Could you check a few things on this model? Use its own coordinates, in mm. Face numbers are marked on the shaded views. A direction names the side the tool comes from. Round coordinates to 2 decimals unless told otherwise and drop trailing zeros. Loops run counter-clockwise (first coordinate to the right, second up) from the corner with the lowest first, then second, coordinate; pieces in that order, holes last. Notation, with made-up numbers: (55, 45.25) -> (60, 45.25) arc R14 cw to (60, 67.25) -> close; hole circle Ø5 at (44, -31.75). An arc over 180 degrees is marked (long way). One line per item, written item: value.
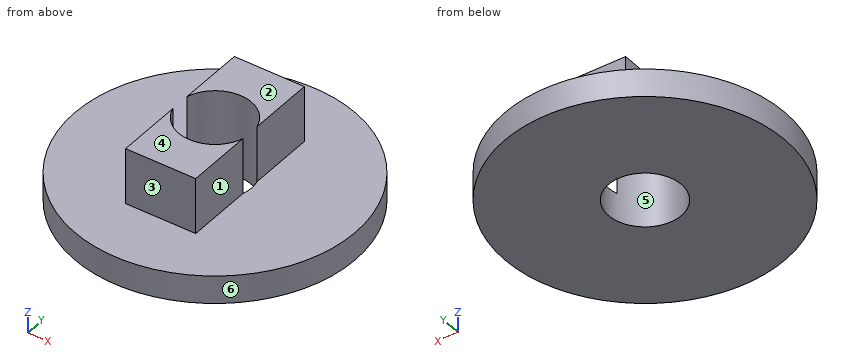
```python
from build123d import *

# Parameters (mm, degrees)
SKETCH1_R                      = 5
BOSS_EXTRUDE1_DEPTH            = 1
SKETCH2_W                      = 2.5
SKETCH2_H                      = 5.454356058
BOSS_EXTRUDE2_DEPTH            = 2
F_2_6_2_6_DIAMETER_HOLE1_D     = 2.6
F_2_6_2_6_DIAMETER_HOLE1_DEPTH = 9
F_2_6_2_6_DIAMETER_HOLE1_TIP   = 0.781118805


with BuildPart() as part:
    # Sketch1 → Boss-Extrude1 (new body)
    with BuildSketch(Plane.XY):
        Circle(SKETCH1_R)
    extrude(amount=BOSS_EXTRUDE1_DEPTH)

    # Sketch2 → Boss-Extrude2 (add)
    with BuildSketch(Plane.XY.offset(1)):
        Rectangle(SKETCH2_W, SKETCH2_H)
    extrude(amount=BOSS_EXTRUDE2_DEPTH)

    # Ø2.6 (2.6) Diameter Hole1
    with Locations(Plane.XY.offset(3)):
        with Locations((0, 0)):
            Hole(F_2_6_2_6_DIAMETER_HOLE1_D / 2, depth=F_2_6_2_6_DIAMETER_HOLE1_DEPTH)
            with Locations((0, 0, -(F_2_6_2_6_DIAMETER_HOLE1_DEPTH + F_2_6_2_6_DIAMETER_HOLE1_TIP / 2))):  # 118° drill point
                Cone(0, F_2_6_2_6_DIAMETER_HOLE1_D / 2, F_2_6_2_6_DIAMETER_HOLE1_TIP, mode=Mode.SUBTRACT)


solid = part.part
```
Item 1: For the marked faces 1 and 2, which set-ups out of +Z, -Z, +X, -X, +Y, -Y let a thin tool reach every point of the face, with its end or its side?
Output:
face 1: +Z, +X, +Y, -Y
face 2: +Z, +X, -X, +Y, -Y
Item 2: If we mould it in two halves opening along Y, with no side actions, what happens to the marked faces 3, 4, 5 and 6? For each: released by +Y, released by -Y, zero draft, split by the parting line, or undercut.
Output:
face 3: released by -Y
face 4: zero draft
face 5: undercut
face 6: split by the parting line
Item 3: If we section it at B-B on z = 2.55: List the corners of the cut face in (x, y) for me, plus the area to 3 significant figures.
Output:
outline: (-1.25, -2.73) -> (1.25, -2.73) -> (1.25, -0.36) arc R1.3 cw to (-1.25, -0.36) -> close; (-1.25, 0.36) arc R1.3 cw to (1.25, 0.36) -> (1.25, 2.73) -> (-1.25, 2.73) -> close
area: 8.37 mm²
Item 4: Will these pins go through, and if not, where does the flat tip stop? pin 1 Ø1.5 at (x, z) = (-3.5, 2.5) entering from +Y; pin 2 Ø1 at (x, z) = (0, 2) entering from +Y; pin 3 Ø1 at (x, y) = (-3.5, 2.5) entering from +Z; pin 4 Ø0.6 at (x, z) = (0.5, 2) entering from -Y.
Output:
pin 1: passes through
pin 2: stops at y = 2.73
pin 3: stops at z = 1
pin 4: stops at y = -2.73
Item 5: If we section it at D-D on z = 0.6: List the corners of the cut face in (x, y) for me.
Output:
outline: circle Ø10 at (0, 0); hole circle Ø2.6 at (0, 0)
Item 6: I need wall thicknesses on line 1 (Y direction, x = 0, z = 1.95); line 2 (Y direction, x = 0, z = 0.9); line 3 (Z direction, x = 2, y = -2.75). Which ranges of each line are inside material? Lowest first, please. Write a range as from..to.
Output:
line 1: y = -2.73..-1.3, 1.3..2.73
line 2: y = -5..-1.3, 1.3..5
line 3: z = 0..1
Item 7: If we section it at A-A on x = 0: List the corners of the cut face in (y, z) for me.
Output:
outline: (-5, 0) -> (-1.3, 0) -> (-1.3, 3) -> (-2.73, 3) -> (-2.73, 1) -> (-5, 1) -> close; (1.3, 0) -> (5, 0) -> (5, 1) -> (2.73, 1) -> (2.73, 3) -> (1.3, 3) -> close
Item 8: If we section it at C-C on y = 0.5: List the corners of the cut face in (x, z) for me.
Output:
outline: (-4.97, 0) -> (-1.2, 0) -> (-1.2, 3) -> (-1.25, 3) -> (-1.25, 1) -> (-4.97, 1) -> close; (1.2, 0) -> (4.97, 0) -> (4.97, 1) -> (1.25, 1) -> (1.25, 3) -> (1.2, 3) -> close
